from build123d import *

# Parameters (mm, degrees)
ESQUISSE1_W             = 45
ESQUISSE1_H             = 10
EXTRUSION1_DEPTH        = 3
ESQUISSE2_R             = 2.6
ENL_V_MAT_EXTRU_1_DEPTH = 3
CONG_1_R                = 5


with BuildPart() as part:
    # Esquisse1 → Extrusion1 (new body)
    with BuildSketch(Plane.XY):
        with Locations((-25.203257042, 6.02306338)):
            Rectangle(ESQUISSE1_W, ESQUISSE1_H)
    extrude(amount=EXTRUSION1_DEPTH)

    # Esquisse2 → Enlèv. mat.-Extru.1 (cut)
    with BuildSketch(Plane.XY.offset(3)):
        with Locations((-40.703257042, 6.02306338)):
            Circle(ESQUISSE2_R)
        with Locations((-9.703257042, 6.02306338)):
            Circle(ESQUISSE2_R)
    extrude(amount=-ENL_V_MAT_EXTRU_1_DEPTH, mode=Mode.SUBTRACT)

    # Congé1
    cong_1_edges = [part.edges().sort_by_distance(p)[0] for p in [
        (-47.703257042, 1.02306338, 1.5),
        (-2.703257042, 1.02306338, 1.5),
        (-2.703257042, 11.02306338, 1.5),
        (-47.703257042, 11.02306338, 1.5),
    ]]
    fillet(cong_1_edges, radius=CONG_1_R - 0.0001)  # a hair under: the kernel refuses the full size


solid = part.part
Read the model definition and answer for the solid it produces. Units are mm, in the model's axes. Round coordinates to 2 decimals unless told otherwise and drop trailing zeros. Order: outer loops, then holes, each group sorted by start corner. A loop starts at its lowest first (then second) coordinate and runs counter-clockwise, first axis right, second up. Notation, with made-up numbers: (3.5, -33) - (46.5, -33) arc R25 cw to (46.5, 4) - close; hole circle Ø1 at (10.25, -28). An arc over 180 degrees is marked (long way). Use one line per item in the form item = value. Start each with the question number.
(1) A flat-ended cylindrical pin translates along its axis: pin 1 Ø1.5 at (y, z) = (4, 1.5) entering from -X. Find the tip coordinate at first contact, or state that the pin passes through.
(2) The part is cut by section B-B (z = 0.75). Count the separate pieces of the cut face and the enclosed holes in it, then the cut area to 3 significant figures.
(3) The part is cut by section A-A (y = 7). Give the vertices of the cut face in (x, z), then the cut area to 3 significant figures.
(4) Find the intervals of material crossed by line 1 along X through (y, z) = (7.25, 2.85); line 2 along X through (y, z) = (3.75, 0.25); line 3 along Y through (x, z) = (-40, 2), in increasing order. Write a range as from..to.
(5) The part is cut by section C-C (y = 4). Give the vertices of the cut face in (x, z), then the cut area to 3 significant figures.
(6) Determine the mould class of faces 1 (the face through (-4.207, 2.449, 1.521)), 2 (the face through (-7.22, 6.8, 1.52)), 3 (the face through (-46.28, 2.53, 1.52)) for opening direction X: +X half, -X half, draft (parallel to the pull), parting line (faces both ways), or undercut.
Checked values:
q1.pin_1 = -47.54
q2.separate_pieces = 1
q2.enclosed_holes = 2
q2.area = 386 mm^2
q3.outline = (-47.61, 0) - (-43.11, 0) - (-43.11, 3) - (-47.61, 3) - close; (-38.29, 0) - (-12.11, 0) - (-12.11, 3) - (-38.29, 3) - close; (-7.29, 0) - (-2.8, 0) - (-2.8, 3) - (-7.29, 3) - close
q3.area = 106 mm^2
q4.line_1 = -47.55..-43, -38.41..-12, -7.41..-2.86
q4.line_2 = -47.16..-41.97, -39.44..-10.97, -8.44..-3.25
q4.line_3 = 1.02..3.52, 8.53..11.02
q5.outline = (-47.28, 0) - (-42.34, 0) - (-42.34, 3) - (-47.28, 3) - close; (-39.07, 0) - (-11.34, 0) - (-11.34, 3) - (-39.07, 3) - close; (-8.07, 0) - (-3.13, 0) - (-3.13, 3) - (-8.07, 3) - close
q5.area = 113 mm^2
q6.face_1 = +X half
q6.face_2 = undercut
q6.face_3 = -X half
